Source: three-view drawing plus pictorial views. Frame: mm from the lowest corner of the part. A direction names the side the tool comes from. Coordinates: 2 decimals unless noted, no trailing zeros. Loops run counter-clockwise (first coordinate to the right, second up) from the corner with the lowest first, then second, coordinate; pieces in that order, holes last. Notation, with made-up numbers: (48, 6) - (53, 6) arc R28 cw to (53, 34) - close; hole circle Ø11 at (56, 65.25). An arc over 180 degrees is marked (long way). Use CSV: the item, a comma, the result in double quotes. Start each with the question number.
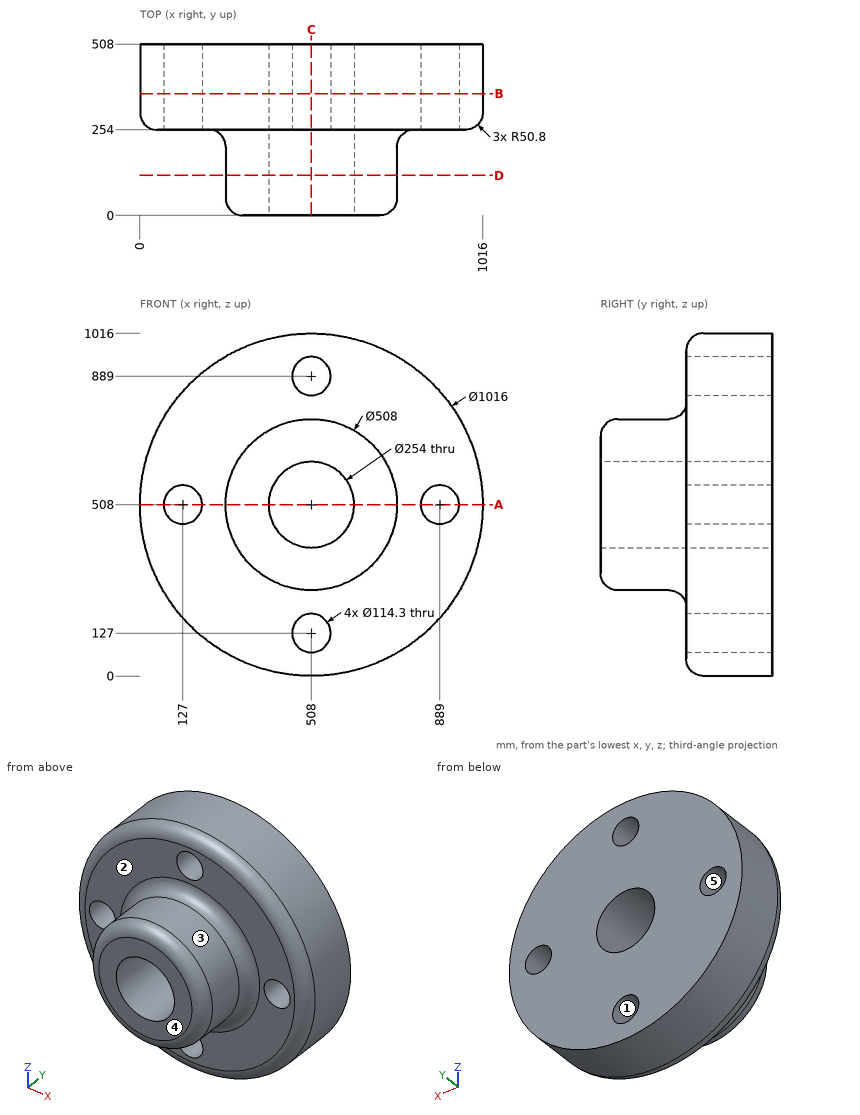
(1) Pin query (flat end, axial travel): pin 1 Ø5 at (x, y) = (594, 299.5) entering from +Z; pin 2 Ø5 at (y, z) = (296, 381.5) entering from +X; pin 3 Ø12 at (y, z) = (331.5, 119.5) entering from +X. Return the tip coordinate at first contact, or that it passes through.
(2) Section A-A on z = 508. Output: boundary loops of the cut face in (x, y).
(3) Ray query, line 1 (X direction, y = 362.5, z = 508); line 2 (X direction, y = 57.5, z = 515.5); line 3 (Y direction, x = 829, z = 447). Return the intervals inside material, ascending. Write a range as [from, to].
(4) Section B-B on y = 361. Output: boundary loops of the cut face in (x, z), plus the area to 3 significant figures.
(5) Section C-C on x = 508. State how many separate pieces and enclosed holes the cut face has, plus the area to 3 significant figures.
(6) Draft query along X for the marked faces 3, 4 and 5. Return one class per face: released by +X, released by -X, zero draft, split by the parting line, or undercut.
(7) Section D-D on y = 118.5. Output: boundary loops of the cut face in (x, z).
(8) Reachability of the marked faces 1 and 2 from +Z, -Z, +X, -X, +Y, -Y: full face, straight path, thin tool, end or side. Return the list, or none.
Solution:
1,pin 1,"stops at z = 1008.87"
1,pin 2,"stops at x = 999.97"
1,pin 3,"stops at x = 842.3"
2,outline,"(0, 304.8) arc R50.8 ccw to (50.8, 254) - (69.85, 254) - (69.85, 508) - (0, 508) - close; (184.15, 254) - (203.2, 254) arc R50.8 cw to (254, 203.2) - (254, 50.8) arc R50.8 ccw to (304.8, 0) - (381, 0) - (381, 508) - (184.15, 508) - close; (635, 0) - (711.2, 0) arc R50.8 ccw to (762, 50.8) - (762, 203.2) arc R50.8 cw to (812.8, 254) - (831.85, 254) - (831.85, 508) - (635, 508) - close; (946.15, 254) - (965.2, 254) arc R50.8 ccw to (1016, 304.8) - (1016, 508) - (946.15, 508) - close"
3,line 1,"x = [0, 69.85], [184.15, 381], [635, 831.85], [946.15, 1016]"
3,line 2,"x = [254.11, 381.22], [634.78, 761.89]"
3,line 3,"y = [254, 508]"
4,outline,"circle Ø1016 at (508, 508); hole circle Ø114.3 at (127, 508); hole circle Ø254 at (508, 508); hole circle Ø114.3 at (508, 127); hole circle Ø114.3 at (508, 889); hole circle Ø114.3 at (889, 508)"
4,area,"719,000 mm²"
5,separate pieces,"4"
5,enclosed holes,"0"
5,area,"199,000 mm²"
6,face 3,"split by the parting line"
6,face 4,"zero draft"
6,face 5,"undercut"
7,outline,"circle Ø508 at (508, 508); hole circle Ø254 at (508, 508)"
8,face 1,"+Y, -Y"
8,face 2,"-Y"
